For this review, use the dimensioned drawing (mm, ordinates from the lowest corner) and the shaded views. A direction names the side the tool comes from. Round coordinates to 2 decimals unless told otherwise and drop trailing zeros. Loops run counter-clockwise (first coordinate to the right, second up) from the corner with the lowest first, then second, coordinate; pieces in that order, holes last. Notation, with made-up numbers: M 22.25,-12 L 67.25,-12 A28 ccw 67.25,15 Z; hole C -32.75,25.25 d6. An arc over 180 degrees is marked long. Answer as a JSON object with one key per item and string values. Group by question number.
Item 1: To check wall thickness, follow line 1 (X direction, y = 30, z = 27.5); line 2 (X direction, y = 36.5, z = 57); line 3 (Y direction, x = 131.5, z = 52). State the ranges of each line that lie inside material, in increasing order.
Item 2: Consider section C-C (x = 113.5). Give the boundary of the cut face in (y, z).
Item 3: Insertion check: P1, Ø4, axis at x = 100, y = 57, coming from the -Z side; P2, Ø1.5, axis at y = 15, z = 70, coming from the -X side; P3, Ø1.5, axis at x = 124.5, z = 38, coming from the -Y side; P4, Ø10, axis at y = 39, z = 34.5, coming from the -X side. Each pin has a flat end and moves straight along its axis. Give the tip position at first contact, or say it passes through.
Item 4: Consider section A-A (z = 40). Give the boundary of the cut face in (x, y).
Item 5: Tool access review of the marked faces 1 and 2: name each direction out of +Z, -Z, +X, -X, +Y, -Y from which nothing blocks a thin tool from reaching the whole face with its end or side.
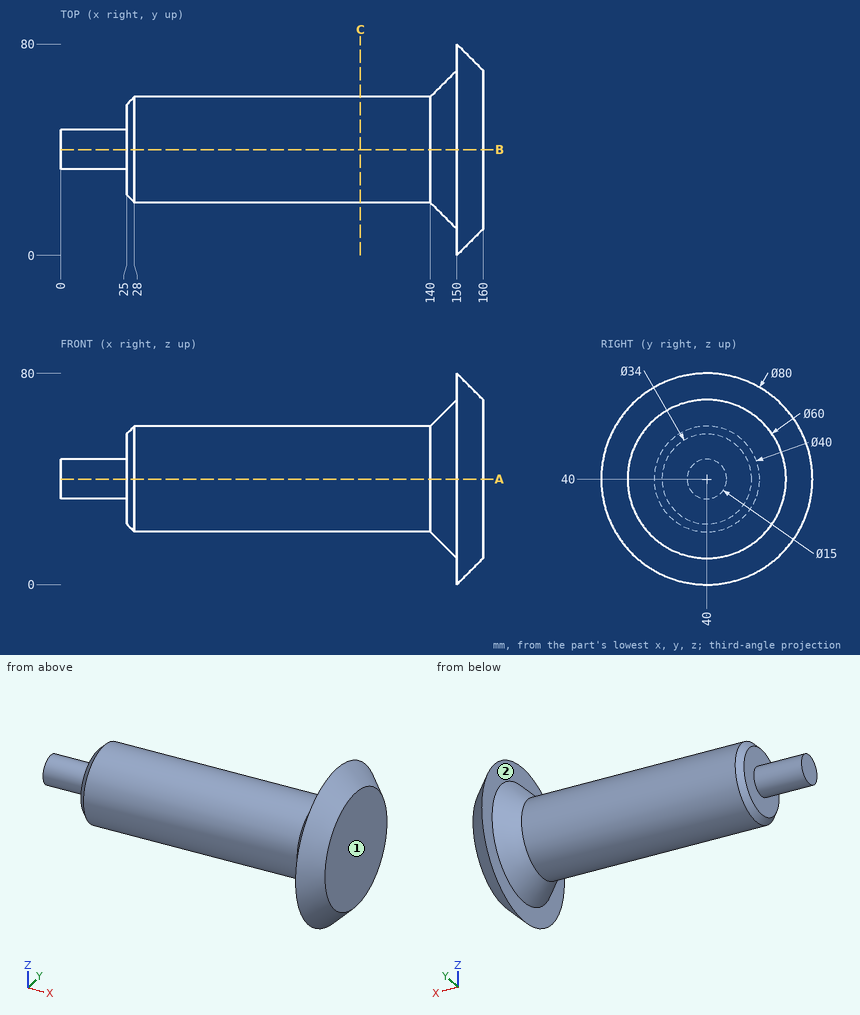
Geometry results:
{
 "1": {"line 1": "x = 25 to 160", "line 2": "x = 25.36 to 160", "line 3": "y = 24 to 56"},
 "2": {"outline": "C 40,40 d40"},
 "3": {"P1": "stops at z = 26.77", "P2": "stops at x = 150", "P3": "stops at y = 20.04", "P4": "stops at x = 0"},
 "4": {"outline": "M 0,32.5 L 25,32.5 L 25,23 L 28,20 L 140,20 L 150,10 L 150,0 L 160,10 L 160,70 L 150,80 L 150,70 L 140,60 L 28,60 L 25,57 L 25,47.5 L 0,47.5 Z"},
 "5": {"face 1": "+Z, -Z, +X, +Y, -Y", "face 2": "-X"}
}
